Verification items for the finished model (mm, model axes). A direction names the side the tool comes from. Give positions to 0.01 mm unless a question says otherwise; leave off trailing zeros. Order: outer loops, then holes, each group sorted by start corner. A loop starts at its lowest first (then second) coordinate and runs counter-clockwise, first axis right, second up. Notation, with made-up numbers: (16.5, 9) -> (64.5, 9) arc R35 cw to (64.5, 45) -> close; hole circle Ø6 at (75.5, -22). An arc over 180 degrees is marked (long way). One line per question, with ' | ' between items. Start each with the question number.
Q1. Section check A-A on x = 26. Record the cut outline in (y, z), plus the area to 3 significant figures.
Q2. Section check D-D on z = -34. Record the cut outline in (x, y), plus the area to 3 significant figures.
Q3. Access from +Z, -Z, +X, -X, +Y, -Y to the whole of each face (thin tool, end or side, straight path). Record for faces 1 (the flat face through (30, 123, -75)), 2 (the flat face through (180, 65, -75)), 3 (the flat face through (0, 104, -61)).
Q4. Material ranges on probe 1 along X at (y, z) = (102.5, -35.5); probe 2 along Y at (x, z) = (176.5, -74); probe 3 along Y at (x, z) = (23, -88), recorded low to high. Write a range as [from, to].
Q5. Go/stop test with flat-tipped pins: pin 1 (0.9 mm diameter, centred on x = 13, y = 182, fed in from +Z); pin 2 (3 mm diameter, centred on x = 77, z = -86, fed in from +Y); pin 3 (16 mm diameter, centred on x = 180.5, z = -89.5, fed in from +Y). Record where each tip stops, or that it passes through.
Q6. Section check C-C on y = 163. Record the cut outline in (x, z), plus the area to 3 significant figures.
Q7. Mould release check, pull along Y, two halves, no side actions. Record for faces 4 (the flat face through (10, 35, -75)), 5 (the flat face through (30, 63, -75)): released by +Y, released by -Y, zero draft, split by the parting line, or undercut.
from build123d import *

# Parameters (mm, degrees)
SKETCH1_W           = 200
SKETCH1_H           = 120
BOSS_EXTRUDE2_DEPTH = 10
SKETCH2_W           = 10
SKETCH2_H           = 110
BOSS_EXTRUDE3_DEPTH = 200
SKETCH3_W           = 70
SKETCH3_H           = 5
BOSS_EXTRUDE4_DEPTH = 20
SKETCH4_W           = 70
SKETCH4_H           = 5
BOSS_EXTRUDE5_DEPTH = 20
SKETCH6_W           = 20
SKETCH6_H           = 3
CUT_EXTRUDE1_DEPTH  = 80
CUT_EXTRUDE2_DEPTH  = 3
SKETCH9_W           = 80
SKETCH9_H           = 3
CUT_EXTRUDE5_DEPTH  = 3
SKETCH10_W          = 20
SKETCH10_H          = 1
CUT_EXTRUDE6_DEPTH  = 70
SKETCH11_W          = 23
SKETCH11_H          = 3
BOSS_EXTRUDE6_DEPTH = 20


with BuildPart() as part:
    # Sketch1 → Boss-Extrude2 (new body)
    with BuildSketch(Plane(origin=(0, 0, 0), x_dir=(1, 0, 0), z_dir=(0, 1, 0))):
        with Locations((100, 60)):
            Rectangle(SKETCH1_W, SKETCH1_H)
    extrude(amount=BOSS_EXTRUDE2_DEPTH)

    # Sketch2 → Boss-Extrude3 (add)
    with BuildSketch(Plane(origin=(0, 10, 0), x_dir=(1, 0, 0), z_dir=(0, 1, 0))):
        with Locations((5, 55)):
            Rectangle(SKETCH2_W, SKETCH2_H)
        Polygon((200, 120), (0, 120), (0, 110), (10, 110), (190, 110), (200, 110), align=None)
        with Locations((195, 55)):
            Rectangle(SKETCH2_W, SKETCH2_H)
    extrude(amount=BOSS_EXTRUDE3_DEPTH)

    # Sketch3 → Boss-Extrude4 (add)
    with BuildSketch(Plane(origin=(10, 0, 0), x_dir=(0, 0, -1), z_dir=(1, 0, 0))):
        with Locations((75, 182.5)):
            Rectangle(SKETCH3_W, SKETCH3_H)
        with Locations((75, 122.5)):
            Rectangle(SKETCH3_W, SKETCH3_H)
        with Locations((75, 62.5)):
            Rectangle(SKETCH3_W, SKETCH3_H)
    extrude(amount=BOSS_EXTRUDE4_DEPTH)

    # Sketch4 → Boss-Extrude5 (add)
    with BuildSketch(Plane.ZY.offset(-190)):
        with Locations((-75, 182.5)):
            Rectangle(SKETCH4_W, SKETCH4_H)
        with Locations((-75, 122.5)):
            Rectangle(SKETCH4_W, SKETCH4_H)
        with Locations((-75, 62.5)):
            Rectangle(SKETCH4_W, SKETCH4_H)
    extrude(amount=BOSS_EXTRUDE5_DEPTH)

    # Sketch6 → Cut-Extrude1 (cut)
    with BuildSketch(Plane.XY.offset(-40)):
        with Locations((20, 182.5)):
            Rectangle(SKETCH6_W, SKETCH6_H)
    extrude(amount=-CUT_EXTRUDE1_DEPTH, mode=Mode.SUBTRACT)

    # Sketch7 → Cut-Extrude2 (cut)
    with BuildSketch(Plane(origin=(10, 0, 0), x_dir=(0, 0, -1), z_dir=(1, 0, 0))):
        Polygon((40, 185), (40, 210), (37, 210), (37, 10), (40, 10), align=None)
    extrude(amount=-CUT_EXTRUDE2_DEPTH, mode=Mode.SUBTRACT)

    # Sketch9 → Cut-Extrude5 (cut)
    with BuildSketch(Plane(origin=(10, 0, 0), x_dir=(0, 0, -1), z_dir=(1, 0, 0))):
        with Locations((80, 182.5)):
            Rectangle(SKETCH9_W, SKETCH9_H)
    extrude(amount=-CUT_EXTRUDE5_DEPTH, mode=Mode.SUBTRACT)

    # Sketch10 → Cut-Extrude6 (cut)
    with BuildSketch(Plane.XY.offset(-40)):
        with Locations((20, 184.5)):
            Rectangle(SKETCH10_W, SKETCH10_H)
        with Locations((20, 180.5)):
            Rectangle(SKETCH10_W, SKETCH10_H)
    extrude(amount=-CUT_EXTRUDE6_DEPTH, mode=Mode.SUBTRACT)

    # Sketch11 → Boss-Extrude6 (add)
    with BuildSketch(Plane(origin=(0, 0, -120), x_dir=(-1, 0, 0), z_dir=(0, 0, -1))):
        with Locations((-18.5, 182.5)):
            Rectangle(SKETCH11_W, SKETCH11_H)
    extrude(amount=-BOSS_EXTRUDE6_DEPTH)


solid = part.part
Filled in:
1) outline: (0, -120) -> (210, -120) -> (210, -110) -> (184, -110) -> (184, -100) -> (181, -100) -> (181, -110) -> (125, -110) -> (125, -40) -> (120, -40) -> (120, -110) -> (65, -110) -> (65, -40) -> (60, -40) -> (60, -110) -> (10, -110) -> (10, 0) -> (0, 0) -> close | area: 3,930 mm²
2) outline: (0, 0) -> (200, 0) -> (200, 210) -> (190, 210) -> (190, 10) -> (10, 10) -> (10, 210) -> (0, 210) -> close | area: 6,000 mm²
3) face 1: +Z, +Y | face 2: +Z | face 3: +Z, -Z, -X, +Y, -Y
4) probe 1: [0, 10], [190, 200] | probe 2: [0, 10], [60, 65], [120, 125], [180, 185] | probe 3: [0, 10], [60, 65], [120, 125]
5) pin 1: z = -100 | pin 2: y = 10 | pin 3: y = 185
6) outline: (0, -120) -> (200, -120) -> (200, 0) -> (190, 0) -> (190, -110) -> (10, -110) -> (10, -40) -> (7, -40) -> (7, -37) -> (10, -37) -> (10, 0) -> (0, 0) -> close | area: 4,190 mm²
7) face 4: undercut | face 5: zero draft
